Verification items for the finished model (mm, model axes). Face numbers are marked on the shaded views. A direction names the side the tool comes from. Give positions to 0.01 mm unless a question says otherwise; leave off trailing zeros. Order: outer loops, then holes, each group sorted by start corner. A loop starts at its lowest first (then second) coordinate and runs counter-clockwise, first axis right, second up. Notation, with made-up numbers: (-23.5, 86) - (11.5, 86) arc R3 ccw to (11.5, 91) - close; hole circle Ø11 at (13, 16). An arc over 180 degrees is marked (long way). Answer as a JSON object with one key per item and string values.
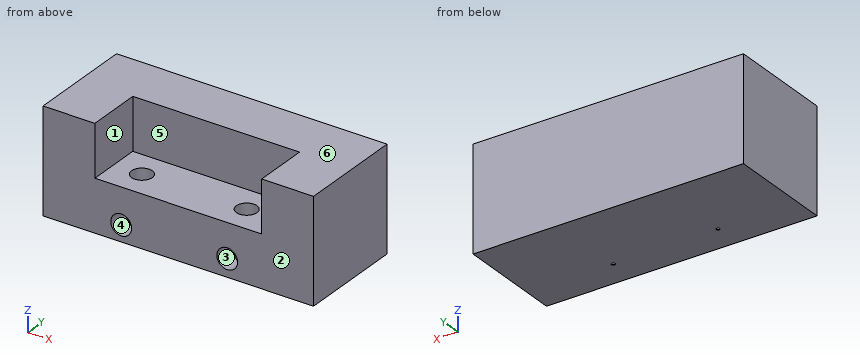
```python
from build123d import *

# Parameters (mm, degrees)
F0_W     = 132.4668824673
F0_H     = 52.4568893015
F1_DEPTH = 25.4
F2_DEPTH = 25.4
F3_T     = -25.4
F5_D     = 10.16
F5_DEPTH = 22.86
F5_TIP   = 3.0523719447
F7_D     = 10.16
F7_DEPTH = 10.16
F7_TIP   = 3.0523719447


with BuildPart() as f1:
    # F0 (on Top) → F1 (new body)
    with BuildSketch(Plane.XY):
        Rectangle(F0_W, F0_H)
    extrude(amount=F1_DEPTH)

    # F2 (add): a face of the model
    f2_faces = [f1.faces().sort_by_distance(p)[0] for p in [
        (0, 0, 0),
    ]]
    extrude(f2_faces, amount=F2_DEPTH)

    # F3
    f3_openings = [f1.faces().sort_by_distance(p)[0] for p in [
        (0, 0, 25.4),
        (0, -26.228445, 0),
    ]]
    offset(amount=F3_T, openings=f3_openings)

    # F5
    with Locations(Plane.XY):
        with Locations((24.2279376835, -12.7), (-27.0736590028, -12.7)):
            Hole(F5_D / 2, depth=F5_DEPTH)
            with Locations((0, 0, -(F5_DEPTH + F5_TIP / 2))):  # 118° drill point
                Cone(0, F5_D / 2, F5_TIP, mode=Mode.SUBTRACT)

    # F7
    with Locations(Plane.XZ.offset(26.2284446508)):
        with Locations((-27.9565155506, -17.5159424543), (23.9731557667, -16.771344468)):
            Hole(F7_D / 2, depth=F7_DEPTH)
            with Locations((0, 0, -(F7_DEPTH + F7_TIP / 2))):  # 118° drill point
                Cone(0, F7_D / 2, F7_TIP, mode=Mode.SUBTRACT)


solid = f1.part
```
(1) Section check D-D (y = -12.7). Record the cut outline in (x, z), then the cut area to 3 significant figures.
Computed values:
{"outline": "(-66.23, -25.4) - (-27.93, -25.4) - (-32.15, -22.86) - (-32.15, 0) - (-40.83, 0) - (-40.83, 25.4) - (-66.23, 25.4) - close; (-26.22, -25.4) - (23.38, -25.4) - (19.15, -22.86) - (19.15, 0) - (-21.99, 0) - (-21.99, -22.86) - close; (25.08, -25.4) - (66.23, -25.4) - (66.23, 25.4) - (40.83, 25.4) - (40.83, 0) - (29.31, 0) - (29.31, -22.86) - close", "area": "4,160 mm²"}
(2) Section check C-C (x = 16). Record the cut outline in (y, z), then the cut area to 3 significant figures.
Computed values:
{"outline": "(-26.23, -25.4) - (26.23, -25.4) - (26.23, 25.4) - (0.83, 25.4) - (0.83, 0) - (-26.23, 0) - close", "area": "1,980 mm²"}
(3) Gauge pin test, flat ends, axial feed: pin 1 Ø12.5 at (x, z) = (11.5, 17) entering from -Y; pin 2 Ø9 at (x, y) = (-27.07, -12.7) entering from +Z. Record the tip position at first contact, or that the pin passes through.
Computed values:
{"pin 1": "stops at y = 0.83", "pin 2": "stops at z = -23.21"}
(4) Section check B-B (y = -5). Record the cut outline in (x, z), then the cut area to 3 significant figures.
Computed values:
{"outline": "(-66.23, -25.4) - (66.23, -25.4) - (66.23, 25.4) - (40.83, 25.4) - (40.83, 0) - (-40.83, 0) - (-40.83, 25.4) - (-66.23, 25.4) - close", "area": "4,650 mm²"}
(5) Material ranges on line 1 along X through (y, z) = (-12.7, -11.75); line 2 along X through (y, z) = (-12, -16); line 3 along Y through (x, z) = (8, 5), recorded low to high. Write a range as [from, to].
Computed values:
{"line 1": "x = [-66.23, -32.15], [-21.99, 19.15], [29.31, 66.23]", "line 2": "x = [-66.23, -32.11], [-22.04, 19.2], [29.26, 66.23]", "line 3": "y = [0.83, 26.23]"}
(6) Release check for a two-part mould opening along Z. For the marked faces 4, 5 and 6 record: pulls with the +Z half, pulls with the -Z half, needs draft (parallel to the pull), parting line crosses it, or undercut.
Computed values:
{"face 4": "undercut", "face 5": "needs draft", "face 6": "pulls with the +Z half"}
(7) Section check A-A (z = 15). Record the cut outline in (x, y), then the cut area to 3 significant figures.
Computed values:
{"outline": "(-66.23, -26.23) - (-40.83, -26.23) - (-40.83, 0.83) - (40.83, 0.83) - (40.83, -26.23) - (66.23, -26.23) - (66.23, 26.23) - (-66.23, 26.23) - close", "area": "4,740 mm²"}
(8) Access from +Z, -Z, +X, -X, +Y, -Y to the whole of each face (thin tool, end or side, straight path). Record for the marked faces 1, 2 and 3.
Computed values:
{"face 1": "+Z, -Y", "face 2": "+Z, -Z, +X, -X, -Y", "face 3": "-Y"}
